```python
from build123d import *

# Parameters (mm, degrees)
F0_W      = 30
F0_H      = 30
F0_R      = 1.6
F1_DEPTH  = 5
F2_DEPTH  = 12
F3_W      = 38
F3_H      = 65
F3_R      = 2
F3_W_2    = 30
F3_H_2    = 5
F4_DEPTH  = 5
F5_DEPTH  = 5
F7_DEPTH  = 20
F8_W      = 20
F8_H      = 5
F9_DEPTH  = 20
F10_R     = 6
F11_DEPTH = 5


with BuildPart() as f1:
    # F0 (on Top) → F1 (new body)
    with BuildSketch(Plane.XY):
        with Locations((-45.2852314338, 17.7588454891)):
            Rectangle(F0_W, F0_H)
        with Locations((-45.2852314338, 12.7588454891)):
            Circle(F0_R, mode=Mode.SUBTRACT)
        with Locations((-49.7852314338, 22.7588454891)):
            Circle(F0_R, mode=Mode.SUBTRACT)
        with Locations((-40.7852314338, 22.7588454891)):
            Circle(F0_R, mode=Mode.SUBTRACT)
    extrude(amount=F1_DEPTH)

    # F2 (add): a face of the model
    f2_faces = [f1.faces().sort_by_distance(p)[0] for p in [
        (-45.2852314338, 32.7588454891, 2.5),
    ]]
    extrude(f2_faces, amount=F2_DEPTH)

    # F3 (on face) → F4 (join)
    with BuildSketch(Plane(origin=(0, 44.7588454891, 0), x_dir=(-1, 0, 0), z_dir=(0, 1, 0))):
        with Locations((48.2852314338, 2.3887734723)):
            Rectangle(F3_W, F3_H)
        with Locations((59.2852314338, -18.1112265277)):
            Circle(F3_R, mode=Mode.SUBTRACT)
        with Locations((45.2852314338, 2.5)):
            Rectangle(F3_W_2, F3_H_2, mode=Mode.SUBTRACT)
        with Locations((59.2852314338, 29.8887734723)):
            Circle(F3_R, mode=Mode.SUBTRACT)
        with Locations((45.2852314338, 2.5)):
            Rectangle(F3_W_2, F3_H_2)
    extrude(amount=F4_DEPTH)

    # F5 (add): a face of the model
    f5_faces = [f1.faces().sort_by_distance(p)[0] for p in [
        (-48.2852314338, 47.2588454891, 34.8887734723),
    ]]
    extrude(f5_faces, amount=F5_DEPTH)

    # F6 (on face) → F7 (join)
    with BuildSketch(Plane.XZ.offset(-44.7588454891)):
        Polygon((-35.2852314338, 39.8887734723), (-55.2852314338, 39.8887734723), (-55.2852314338, 34.8887734723), (-45.2852314338, 34.8887734723), (-35.2852314338, 34.8887734723), align=None)
    extrude(amount=F7_DEPTH)

    # F8 (on face) → F9 (join)
    with BuildSketch(Plane.XY.offset(39.8887734723)):
        with Locations((-45.2852314338, 27.2588454891)):
            Rectangle(F8_W, F8_H)
    extrude(amount=F9_DEPTH)

    # F10 (on face) → F11 (cut)
    with BuildSketch(Plane(origin=(0, 29.7588454891, 0), x_dir=(-1, 0, 0), z_dir=(0, 1, 0))):
        with Locations((45.2852314338, 49.8887734723)):
            Circle(F10_R)
    extrude(amount=-F11_DEPTH, mode=Mode.SUBTRACT)


solid = f1.part
```
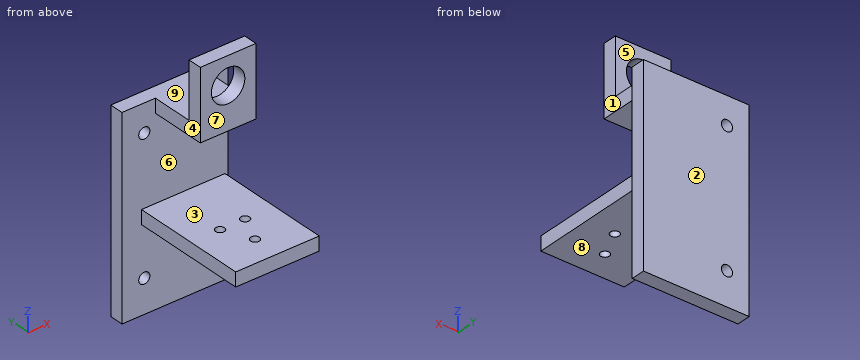
Source: CAD feature listing. Evaluate the final solid. Frame: model axes, mm. Face numbers are marked on the shaded views. A direction names the side the tool comes from. Round coordinates to 2 decimals unless told otherwise and drop trailing zeros. Loops run counter-clockwise (first coordinate to the right, second up) from the corner with the lowest first, then second, coordinate; pieces in that order, holes last.
1. Mould query, pull axis Z, two halves, no side actions, for the marked faces 6, 7, 8 and 9. Classes: released by +Z, released by -Z, zero draft, split by the parting line, or undercut.
2. Section query C-C on z = 47.5. Output: boundary loops of the cut face in (x, y).
3. Ray query, L1, parallel to Z at x = -45.5, y = 26; L2, parallel to Z at x = -37.5, y = 43; L3, parallel to X at y = 22, z = 1.5. Return the intervals inside material, ascending.
4. Access query for the marked faces 1, 2, 3, 4 and 5. Directions: +Z, -Z, +X, -X, +Y, -Y. A direction counts if a zero-diameter tool reaches every point of the face in a straight line with its end or side. Return the directions, or none.
5. Section query B-B on x = -52.5. Output: boundary loops of the cut face in (y, z).
6. Section query D-D on y = 42.5. Output: boundary loops of the cut face in (x, z), and give its area (3 significant figures).
7. Contact query for flat-ended pins moving along their axis: pin 1 (1.5 mm diameter, centred on x = -52, y = 12, fed in from -Z); pin 2 (4 mm diameter, centred on y = 24.5, z = 44.5, fed in from -X); pin 3 (2 mm diameter, centred on x = -39, z = 31.5, fed in from -Y). Output: stop coordinate, or through.
8. Section query A-A on y = 28.5. Output: boundary loops of the cut face in (x, z), and give its area (3 significant figures).
Answers below:
1. face 6: undercut
1. face 7: zero draft
1. face 8: released by -Z
1. face 9: released by +Z
2. outline: (-55.29, 24.76) - (-50.79, 24.76) - (-50.79, 29.76) - (-55.29, 29.76) - close; (-39.78, 24.76) - (-35.29, 24.76) - (-35.29, 29.76) - (-39.78, 29.76) - close
3. L1: z = 0 to 5, 34.89 to 43.89, 55.88 to 59.89
3. L2: z = 0 to 5, 34.89 to 39.89
3. L3: x = -60.29 to -51.19, -48.38 to -42.19, -39.38 to -30.29
4. face 1: +Z, +X, -Y
4. face 2: +Z, -Z, +X, -X, +Y
4. face 3: +X, -X, -Y
4. face 4: +Z, -X, -Y
4. face 5: +Z, +X, -X, +Y
5. outline: (2.76, 0) - (44.76, 0) - (44.76, -30.11) - (49.76, -30.11) - (49.76, 39.89) - (29.76, 39.89) - (29.76, 59.89) - (24.76, 59.89) - (24.76, 34.89) - (44.76, 34.89) - (44.76, 5) - (2.76, 5) - close
6. outline: (-60.29, 0) - (-30.29, 0) - (-30.29, 5) - (-60.29, 5) - close; (-55.29, 34.89) - (-35.29, 34.89) - (-35.29, 39.89) - (-55.29, 39.89) - close
6. area: 250 mm2
7. pin 1: stops at z = 0
7. pin 2: stops at x = -55.29
7. pin 3: stops at y = 44.76
8. outline: (-60.29, 0) - (-30.29, 0) - (-30.29, 5) - (-60.29, 5) - close; (-55.29, 34.89) - (-35.29, 34.89) - (-35.29, 59.89) - (-55.29, 59.89) - close; hole circle Ø12 at (-45.29, 49.89)
8. area: 537 mm2
